Source: CAD feature listing. Evaluate the final solid. Frame: model axes, mm. A direction names the side the tool comes from. Round coordinates to 2 decimals unless told otherwise and drop trailing zeros. Order: outer loops, then holes, each group sorted by start corner. A loop starts at its lowest first (then second) coordinate and runs counter-clockwise, first axis right, second up. Notation, with made-up numbers: (24.25, 10) -> (29.25, 10) arc R29 ccw to (29.25, 31) -> close; hole circle Ø6 at (39.5, 14.25). An arc over 180 degrees is marked (long way). Answer as CSV lines item,"result". Start each with the question number.
(1) Set-up query: faces 4 (the cylindrical face through (-27.397, -6.822, 3.479)), 5 (the flat face through (-27.5, 0, 1)), 6 (the flat face through (0, 7.5, 1)). Return all of +Z, -Z, +X, -X, +Y, -Y with unobstructed straight access to the full face (end or side cutting, diameter ignored); none if empty.
(2) Section query A-A (z = 3.8). Output: boundary loops of the cut face in (x, y), plus the area to 3 significant figures.
(3) Contact query for a flat-ended pin moving along its axis: P1, Ø1.5, axis at y = 5.5, z = 3.5, coming from the -X side. Output: stop coordinate, or through.
(4) Line query: line 1 along Y through (x, z) = (-24.5, 0.7); line 2 along Y through (x, z) = (24.5, 3); line 3 along Y through (x, z) = (7, 0.4). Output: solid intervals per line, ascending. Write a range as from..to.
(5) Pull-direction query (Y, two-part tool) for faces 1 (the flat face through (0, 10.5, 1)), 2 (the flat face through (23, 6, 5)), 3 (the cylindrical face through (22.96, -0.16, 1.01)); classes: +Y half, -Y half, draft (parallel to the pull), parting line (faces both ways), or undercut.
(6) Section query B-B (x = 24.5). Output: boundary loops of the cut face in (y, z), plus the area to 3 significant figures.
(7) Section query D-D (x = 13). Output: boundary loops of the cut face in (y, z).
(8) Section query C-C (y = 0). Output: boundary loops of the cut face in (x, z).
```python
from build123d import *

# Parameters (mm, degrees)
SKETCH_W        = 55
SKETCH_H        = 21
PAD_DEPTH       = 2
SKETCH001_R     = 1.45
POCKET_DEPTH    = 2.001
SKETCH002_R     = 2.9
SKETCH002_R_2   = 1.45
PAD001_DEPTH    = 3
POCKET001_DEPTH = 2.001


with BuildPart() as part:
    # Sketch → Pad (new body)
    with BuildSketch(Plane.XY):
        Rectangle(SKETCH_W, SKETCH_H)
    extrude(amount=PAD_DEPTH)

    # Sketch001 (on Face6 of Pad) → Pocket (cut, through all)
    with BuildSketch(Plane.XY.offset(2)):
        with Locations((-24.5, 6.95)):
            Circle(SKETCH001_R)
        with Locations((24.5, 6.95)):
            Circle(SKETCH001_R)
        with Locations((24.5, -6.95)):
            Circle(SKETCH001_R)
        with Locations((-24.5, -6.95)):
            Circle(SKETCH001_R)
    extrude(amount=-POCKET_DEPTH, mode=Mode.SUBTRACT)

    # Sketch002 (on Face5 of Pocket) → Pad001 (join)
    with BuildSketch(Plane.XY.offset(2)):
        with Locations((-24.5, 6.95)):
            Circle(SKETCH002_R)
        with Locations((-24.5, 6.95)):
            Circle(SKETCH002_R_2, mode=Mode.SUBTRACT)
        with Locations((24.5, 6.95)):
            Circle(SKETCH002_R)
        with Locations((24.5, 6.95)):
            Circle(SKETCH002_R_2, mode=Mode.SUBTRACT)
        with Locations((24.5, -6.95)):
            Circle(SKETCH002_R)
        with Locations((24.5, -6.95)):
            Circle(SKETCH002_R_2, mode=Mode.SUBTRACT)
        with Locations((-24.5, -6.95)):
            Circle(SKETCH002_R)
        with Locations((-24.5, -6.95)):
            Circle(SKETCH002_R_2, mode=Mode.SUBTRACT)
    extrude(amount=PAD001_DEPTH)

    # Sketch003 (on Face5 of Pad001) → Pocket001 (cut, through all)
    with BuildSketch(Plane.XY.offset(2)):
        with BuildLine():
            ThreePointArc((-15.459811, 7.5), (-22.959811, 0), (-15.459811, -7.5))
            Line((-15.459811, -7.5), (15.459811, -7.5))
            ThreePointArc((15.459811, -7.5), (22.959811, 0), (15.459811, 7.5))
            Line((15.459811, 7.5), (-15.459811, 7.5))
        make_face()
    extrude(amount=-POCKET001_DEPTH, mode=Mode.SUBTRACT)


solid = part.part
```
Answer block:
1,face 4,"+Z"
1,face 5,"+Z, -Z, -X, +Y, -Y"
1,face 6,"+Z, -Z"
2,outline,"circle Ø5.8 at (-24.5, -6.95); circle Ø5.8 at (-24.5, 6.95); circle Ø5.8 at (24.5, -6.95); circle Ø5.8 at (24.5, 6.95); hole circle Ø2.9 at (-24.5, -6.95); hole circle Ø2.9 at (-24.5, 6.95); hole circle Ø2.9 at (24.5, -6.95); hole circle Ø2.9 at (24.5, 6.95)"
2,area,"79.3 mm2"
3,P1,"x = -27.31"
4,line 1,"-10.5..-8.4, -5.5..5.5, 8.4..10.5"
4,line 2,"-9.85..-8.4, -5.5..-4.05, 4.05..5.5, 8.4..9.85"
4,line 3,"-10.5..-7.5, 7.5..10.5"
5,face 1,"+Y half"
5,face 2,"draft"
5,face 3,"undercut"
6,outline,"(-10.5, 0) -> (-8.4, 0) -> (-8.4, 5) -> (-9.85, 5) -> (-9.85, 2) -> (-10.5, 2) -> close; (-5.5, 0) -> (5.5, 0) -> (5.5, 5) -> (4.05, 5) -> (4.05, 2) -> (-4.05, 2) -> (-4.05, 5) -> (-5.5, 5) -> close; (8.4, 0) -> (10.5, 0) -> (10.5, 2) -> (9.85, 2) -> (9.85, 5) -> (8.4, 5) -> close"
6,area,"47.8 mm2"
7,outline,"(-10.5, 0) -> (-7.5, 0) -> (-7.5, 2) -> (-10.5, 2) -> close; (7.5, 0) -> (10.5, 0) -> (10.5, 2) -> (7.5, 2) -> close"
8,outline,"(-27.5, 0) -> (-22.96, 0) -> (-22.96, 2) -> (-27.5, 2) -> close; (22.96, 0) -> (27.5, 0) -> (27.5, 2) -> (22.96, 2) -> close"
